```python
from build123d import *
from build123d.topology import SkipClean

# Parameters (mm, degrees)
SKETCH2_W                      = 63.5
SKETCH2_H                      = 63.5
BOSS_EXTRUDE1_DEPTH            = 80
CUT_EXTRUDE1_REACH             = 93.739
SKETCH4_R                      = 14.2875
CUT_EXTRUDE2_DEPTH             = 3.81
CUT_EXTRUDE3_DEPTH             = 62.22
CUT_EXTRUDE4_REACH             = 93.739
CUT_EXTRUDE4_DIRECTION_2_REACH = 93.739
FILLET2_R                      = 2.54
SKETCH9_W                      = 5
SKETCH9_H                      = 80
BOSS_EXTRUDE2_DEPTH            = 35
SKETCH10_R                     = 2.75
CUT_EXTRUDE6_DEPTH             = 119.642846392
CUT_EXTRUDE7_REACH             = 110.92
SKETCH11_R                     = 3
SKETCH12_W                     = 40
SKETCH12_H                     = 80
BOSS_EXTRUDE3_DEPTH            = 15
SKETCH13_R                     = 3
CUT_EXTRUDE8_DEPTH             = 10
FILLET3_R                      = 3.175
FILLET4_DEPTH                  = 80


with BuildPart() as part:
    # Sketch2 → Boss-Extrude1 (new body)
    with BuildSketch(Plane(origin=(0, 0, 0), x_dir=(1, 0, 0), z_dir=(0, 1, 0))):
        Rectangle(SKETCH2_W, SKETCH2_H)
    extrude(amount=BOSS_EXTRUDE1_DEPTH)

    # Sketch3 → Cut-Extrude1 (cut, up to next)
    with BuildSketch(Plane(origin=(0, 80, 0), x_dir=(1, 0, 0), z_dir=(0, 1, 0)), mode=Mode.PRIVATE) as cut_extrude1_sk1:
        with BuildLine():
            Line((9.525, 0), (14.2875, 0))
            ThreePointArc((14.2875, 0), (0, -14.2875), (-14.2875, 0))
            Line((-14.2875, 0), (-9.525, 0))
            ThreePointArc((-9.525, 0), (0, 9.525), (9.525, 0))
        make_face()
    cut_extrude1_tool1 = extrude(cut_extrude1_sk1.sketch, amount=-CUT_EXTRUDE1_REACH, mode=Mode.PRIVATE) & part.part
    add(cut_extrude1_tool1.solids().sort_by_distance((0, 80, 2.954161))[0], mode=Mode.SUBTRACT)

    # Sketch4 → Cut-Extrude2 (cut)
    with BuildSketch(Plane(origin=(0, 80, 0), x_dir=(1, 0, 0), z_dir=(0, 1, 0))):
        with Locations(Location((0, 0, 0), (0, 0, 270))):
            Circle(SKETCH4_R)
    extrude(amount=-CUT_EXTRUDE2_DEPTH, mode=Mode.SUBTRACT)

    # Sketch6 → Cut-Extrude3 (cut)
    with BuildSketch(Plane(origin=(0, 71.11, 0), x_dir=(1, 0, 0), z_dir=(0, 1, 0))):
        with BuildLine():
            Line((9.525, 0), (19.05, 31.75))
            Line((19.05, 31.75), (-19.05, 31.75))
            Line((-19.05, 31.75), (-9.525, 0))
            ThreePointArc((-9.525, 0), (0, 9.525), (9.525, 0))
        make_face()
    extrude(amount=-CUT_EXTRUDE3_DEPTH, mode=Mode.SUBTRACT)

    # Cut-Extrude4: up to this plane
    with SkipClean():  # the faces are left unmerged after this step: merging them gives an invalid solid
        cut_extrude4_end = Plane(origin=(-9.525, -49.595085442, 0), z_dir=(-0.9578262852211514, 0, 0.2873478855663456))
        # Sketch7 → Cut-Extrude4 (cut, up to the surface)
        with BuildSketch(Plane(origin=(0, 0, 0), x_dir=(0, 0, -1), z_dir=(1, 0, 0)), mode=Mode.PRIVATE) as cut_extrude4_sk1:
            Polygon((0, 8.89), (31.75, 8.89), (0, 0), align=None)
        cut_extrude4_tool1 = split(extrude(cut_extrude4_sk1.sketch, amount=-CUT_EXTRUDE4_REACH, mode=Mode.PRIVATE), bisect_by=cut_extrude4_end, keep=Keep.BOTH, mode=Mode.PRIVATE)
        add(cut_extrude4_tool1.solids().sort_by_distance((0, 5.926667, -10.583333))[0], mode=Mode.SUBTRACT)

    # Cut-Extrude4 direction 2: up to this plane
    cut_extrude4_direction_2_end = Plane(origin=(9.525, -49.595085442, 0), z_dir=(0.9578262852211514, 0, 0.2873478855663456))
    # Sketch7 → Cut-Extrude4 direction 2 (cut, up to the surface)
    with BuildSketch(Plane(origin=(0, 0, 0), x_dir=(0, 0, -1), z_dir=(1, 0, 0)), mode=Mode.PRIVATE) as cut_extrude4_direction_2_sk1:
        Polygon((0, 8.89), (31.75, 8.89), (0, 0), align=None)
    cut_extrude4_direction_2_tool1 = split(extrude(cut_extrude4_direction_2_sk1.sketch, amount=CUT_EXTRUDE4_DIRECTION_2_REACH, mode=Mode.PRIVATE), bisect_by=cut_extrude4_direction_2_end, keep=Keep.BOTH, mode=Mode.PRIVATE)
    add(cut_extrude4_direction_2_tool1.solids().sort_by_distance((0, 5.926667, -10.583333))[0], mode=Mode.SUBTRACT)

    # Fillet2
    # the kernel refuses this fillet: 2.54 mm, written as the material it adds along each edge
    with BuildSketch(Plane(origin=(7.700340927, 71.11, 6.082196911), x_dir=(-0.9578262852211513, 0, -0.2873478855663455), z_dir=(0.28734788556634555, 0, -0.9578262852211513))) as fillet2_piece_1_section:
        with BuildLine():
            CenterArc((FILLET2_R, -FILLET2_R), FILLET2_R, 90, 90)
            Line((0, -FILLET2_R), (0, 0))
            Line((0, 0), (FILLET2_R, 0))
        make_face()
    fillet2_piece_1 = extrude(amount=45.847973166, mode=Mode.PRIVATE)
    fillet2_piece_1 = split(fillet2_piece_1, bisect_by=Plane(origin=(7.700340927, 71.11, -31.75), z_dir=(0, 0, 1)), keep=Keep.TOP, mode=Mode.PRIVATE)
    fillet2_piece_1 = fillet2_piece_1 - Plane(origin=(0, 71.11, 0), x_dir=(-1, 0, 0), z_dir=(0, 1, 0)) * Cylinder(9.525, 102, mode=Mode.PRIVATE)
    fillet2_piece_1 = split(fillet2_piece_1, bisect_by=Plane(origin=(7.700340927, 71.11, 0), z_dir=(0, 0, -1)), keep=Keep.TOP, mode=Mode.PRIVATE)
    add(fillet2_piece_1)
    with BuildSketch(Plane(origin=(-20.874659073, 71.11, -37.832196911), x_dir=(0, -1, 0), z_dir=(0.28734788556634555, 0, 0.9578262852211513))) as fillet2_piece_2_section:
        with BuildLine():
            CenterArc((FILLET2_R, FILLET2_R), FILLET2_R, 180, 90)
            Line((0, FILLET2_R), (0, 0))
            Line((0, 0), (FILLET2_R, 0))
        make_face()
    fillet2_piece_2 = extrude(amount=45.847973166, mode=Mode.PRIVATE)
    fillet2_piece_2 = split(fillet2_piece_2, bisect_by=Plane(origin=(-20.874659073, 71.11, -31.75), z_dir=(0, 0, 1)), keep=Keep.TOP, mode=Mode.PRIVATE)
    fillet2_piece_2 = split(fillet2_piece_2, bisect_by=Plane(origin=(-20.874659073, 71.11, 0), z_dir=(0, 0, -1)), keep=Keep.TOP, mode=Mode.PRIVATE)
    fillet2_piece_2 = fillet2_piece_2 - Plane(origin=(0, 71.11, 0), x_dir=(-1, 0, 0), z_dir=(0, 1, 0)) * Cylinder(9.525, 102, mode=Mode.PRIVATE)
    add(fillet2_piece_2)
    with BuildSketch(Plane(origin=(-20.954648619, 10.667672044, -38.098828729), x_dir=(0.9607141016314922, 0.07483307171461691, -0.2672609704093551), z_dir=(0.2775399339309484, -0.2590372716688848, 0.9251331131031606))) as fillet2_piece_3_section:
        with BuildLine():
            CenterArc((FILLET2_R * 1.08072615035, FILLET2_R), FILLET2_R, 175.556407911, 94.443592089)
            Line((FILLET2_R * 0.0837320564804, FILLET2_R * 1.07747758898), (0, 0))
            Line((0, 0), (FILLET2_R * 1.08072615035, 0))
        make_face()
    fillet2_piece_3 = extrude(amount=52.848435405, mode=Mode.PRIVATE)
    fillet2_piece_3 = split(fillet2_piece_3, bisect_by=Plane(origin=(-20.954648619, 10.667672044, -31.75), z_dir=(0, 0, 1)), keep=Keep.TOP, mode=Mode.PRIVATE)
    fillet2_piece_3 = fillet2_piece_3 - Plane(origin=(0, 10.667672044, 0), x_dir=(-1, 0, 0), z_dir=(0, 1, 0)) * Cylinder(9.525, 117, mode=Mode.PRIVATE)
    fillet2_piece_3 = split(fillet2_piece_3, bisect_by=Plane(origin=(-20.954648619, 10.667672044, 0), z_dir=(0, 0, -1)), keep=Keep.TOP, mode=Mode.PRIVATE)
    add(fillet2_piece_3)
    with BuildSketch(Plane(origin=(20.954648619, 10.667672044, -38.098828729), x_dir=(-0.9607141016314922, 0.07483307171461691, -0.2672609704093551), z_dir=(-0.2775399339309484, -0.2590372716688848, 0.9251331131031606))) as fillet2_piece_4_section:
        with BuildLine():
            CenterArc((FILLET2_R * 1.08072615035, -FILLET2_R), FILLET2_R, 90, 94.443592089)
            Line((FILLET2_R * 0.0837320564804, -FILLET2_R * 1.07747758898), (0, 0))
            Line((0, 0), (FILLET2_R * 1.08072615035, 0))
        make_face()
    fillet2_piece_4 = extrude(amount=52.848435405, mode=Mode.PRIVATE)
    fillet2_piece_4 = split(fillet2_piece_4, bisect_by=Plane(origin=(20.954648619, 10.667672044, -31.75), z_dir=(0, 0, 1)), keep=Keep.TOP, mode=Mode.PRIVATE)
    fillet2_piece_4 = fillet2_piece_4 - Plane(origin=(0, 10.667672044, 0), x_dir=(-1, 0, 0), z_dir=(0, 1, 0)) * Cylinder(9.525, 117, mode=Mode.PRIVATE)
    fillet2_piece_4 = split(fillet2_piece_4, bisect_by=Plane(origin=(20.954648619, 10.667672044, 0), z_dir=(0, 0, -1)), keep=Keep.TOP, mode=Mode.PRIVATE)
    add(fillet2_piece_4)

    # Sketch9 → Boss-Extrude2 (add)
    with BuildSketch(Plane.XY.offset(31.75)):
        with Locations((-22.5, 40)):
            Rectangle(SKETCH9_W, SKETCH9_H)
        with Locations((22.5, 40)):
            Rectangle(SKETCH9_W, SKETCH9_H)
    extrude(amount=BOSS_EXTRUDE2_DEPTH)

    # Sketch10 → Cut-Extrude6 (cut, through all)
    with BuildSketch(Plane.ZY.offset(25)):
        with Locations(Location((56.75, 70, 0), (0, 0, 270))):
            Circle(SKETCH10_R)
        with Locations(Location((56.75, 10, 0), (0, 0, 270))):
            Circle(SKETCH10_R)
    extrude(amount=-CUT_EXTRUDE6_DEPTH, mode=Mode.SUBTRACT)

    # Sketch11 → Cut-Extrude7 (cut, up to next)
    with BuildSketch(Plane.XZ, mode=Mode.PRIVATE) as cut_extrude7_sk1:
        with Locations(Location((26.042742751, -26.042742751, 0), (0, 0, 270))):
            Circle(SKETCH11_R)
    cut_extrude7_tool1 = extrude(cut_extrude7_sk1.sketch, amount=-CUT_EXTRUDE7_REACH, mode=Mode.PRIVATE) & part.part
    # Sketch11 → Cut-Extrude7 (cut, up to next)
    with BuildSketch(Plane.XZ, mode=Mode.PRIVATE) as cut_extrude7_sk2:
        with Locations(Location((26.042742751, 26.042742751, 0), (0, 0, 270))):
            Circle(SKETCH11_R)
    cut_extrude7_tool2 = extrude(cut_extrude7_sk2.sketch, amount=-CUT_EXTRUDE7_REACH, mode=Mode.PRIVATE) & part.part
    # Sketch11 → Cut-Extrude7 (cut, up to next)
    with BuildSketch(Plane.XZ, mode=Mode.PRIVATE) as cut_extrude7_sk3:
        with Locations(Location((-26.042742751, -26.042742751, 0), (0, 0, 270))):
            Circle(SKETCH11_R)
    cut_extrude7_tool3 = extrude(cut_extrude7_sk3.sketch, amount=-CUT_EXTRUDE7_REACH, mode=Mode.PRIVATE) & part.part
    # Sketch11 → Cut-Extrude7 (cut, up to next)
    with BuildSketch(Plane.XZ, mode=Mode.PRIVATE) as cut_extrude7_sk4:
        with Locations(Location((-26.042742751, 26.042742751, 0), (0, 0, 270))):
            Circle(SKETCH11_R)
    cut_extrude7_tool4 = extrude(cut_extrude7_sk4.sketch, amount=-CUT_EXTRUDE7_REACH, mode=Mode.PRIVATE) & part.part
    add(cut_extrude7_tool1.solids().sort_by_distance((26.042743, 0, -26.042743))[0], mode=Mode.SUBTRACT)
    add(cut_extrude7_tool2.solids().sort_by_distance((26.042743, 0, 26.042743))[0], mode=Mode.SUBTRACT)
    add(cut_extrude7_tool3.solids().sort_by_distance((-26.042743, 0, -26.042743))[0], mode=Mode.SUBTRACT)
    add(cut_extrude7_tool4.solids().sort_by_distance((-26.042743, 0, 26.042743))[0], mode=Mode.SUBTRACT)

    # Sketch12 → Boss-Extrude3 (add)
    with BuildSketch(Plane.XY.offset(31.75)):
        with Locations((0, 40)):
            Rectangle(SKETCH12_W, SKETCH12_H)
    extrude(amount=BOSS_EXTRUDE3_DEPTH)

    # Sketch13 → Cut-Extrude8 (cut)
    with BuildSketch(Plane(origin=(0, 0, -31.75), x_dir=(-1, 0, 0), z_dir=(0, 0, -1))):
        with Locations((-18.75, 75)):
            Circle(SKETCH13_R)
        with Locations(Location((18.75, 75, 0), (0, 0, 180))):
            Circle(SKETCH13_R)
        with Locations((18.75, 5)):
            Circle(SKETCH13_R)
        with Locations(Location((-18.75, 5, 0), (0, 0, 180))):
            Circle(SKETCH13_R)
    extrude(amount=-CUT_EXTRUDE8_DEPTH, mode=Mode.SUBTRACT)

    # Fillet3
    fillet3_edges = [part.edges().sort_by_distance(p)[0] for p in [
        (31.75, 40, 31.75),
        (-31.75, 40, 31.75),
        (-31.75, 40, -31.75),
        (31.75, 40, -31.75),
    ]]
    fillet(fillet3_edges, radius=FILLET3_R)

    # Fillet4: read off the stored shape, not the designer's step
    # Fillet4 outline → Fillet4 (add)
    with BuildSketch(Plane(origin=(0, 0, 0), x_dir=(1, 0, 0), z_dir=(0, 1, 0))):
        with BuildLine():
            Line((25, -31.75), (25, -36.624844719))
            ThreePointArc((25, -36.624844719), (26.168694859, -33.412197692), (29.128440367, -31.701392291))
            ThreePointArc((29.128440367, -31.701392291), (28.852785416, -31.737824728), (28.575, -31.75))
            Line((28.575, -31.75), (25, -31.75))
        make_face()
        with BuildLine():
            ThreePointArc((-28.575, -31.75), (-28.852785416, -31.737824728), (-29.128440367, -31.701392291))
            ThreePointArc((-29.128440367, -31.701392291), (-26.168694859, -33.412197692), (-25, -36.624844719))
            Line((-25, -36.624844719), (-25, -31.75))
            Line((-25, -31.75), (-28.575, -31.75))
        make_face()
    extrude(amount=FILLET4_DEPTH)


solid = part.part
```
The listing builds one solid part. Answer for the finished solid, in the listing's coordinates (mm). A direction names the side the tool comes from. Coordinates: 2 decimals unless noted, no trailing zeros. Write each loop counter-clockwise with the first axis right and the second up, starting at its lowest first coordinate (ties: lowest second). Pieces come first, ordered by that corner, then holes.
Q1. The mould has two halves that part along X. Classify faces 6 (the cylindrical face through (26.137, 39.44, 33.45)), 7 (the flat face through (-23, 41, 66.75)), 8 (the flat face through (19, 75, -21.75)), 9 (the cylindrical face through (-31.03, 40.56, 30.59)): released by +X, released by -X, zero draft, split by the parting line, or undercut.
Returned:
face 6: released by +X
face 7: zero draft
face 8: undercut
face 9: released by -X
Q2. Section D-D, the plane z = 43.5 is taken. Write down the section's boundary in (x, y).
Returned:
outline: (-25, 0) - (25, 0) - (25, 80) - (-25, 80) - close
Q3. Find the intervals of material crossed by line 1 along Y through (x, z) = (18.75, -28.75); line 2 along Z through (x, y) = (-23, 10); line 3 along Z through (x, y) = (-24.5, 47.5), in increasing order.
Returned:
line 1: y = 0 to 2, 8 to 72, 78 to 80
line 2: z = -31.75 to 54, 59.5 to 66.75
line 3: z = -31.75 to -28.62, -23.47 to 23.47, 28.62 to 66.75
Q4. Given P1, Ø6, axis at y = 35, z = 54.5, coming from the +X side; P2, Ø5, axis at x = -26.04, z = -26.04, coming from the +Y side; P3, Ø1.4, axis at x = -12.5, y = 24.5, coming from the +Z side; P4, Ø3, axis at x = 18, y = 74.5, coming from the -Z side, each flat-ended and moving along its own axis, determine where each tip first touches the part or whether it passes through.
Returned:
P1: stops at x = 25
P2: passes through
P3: stops at z = 46.75
P4: stops at z = -21.75
Q5. Section B-B, the plane y = 47.5 is taken. Give the number of separate pieces and of enclosed holes in the cut face, then the cut area to 3 significant figures.
Returned:
separate pieces: 1
enclosed holes: 4
area: 3,640 mm2
Q6. Section A-A, the plane z = 56.75 is taken. Write down the section's boundary in (x, y), then the cut area to 3 significant figures.
Returned:
outline: (-25, 0) - (-20, 0) - (-20, 7.25) - (-25, 7.25) - close; (-25, 12.75) - (-20, 12.75) - (-20, 67.25) - (-25, 67.25) - close; (-25, 72.75) - (-20, 72.75) - (-20, 80) - (-25, 80) - close; (20, 0) - (25, 0) - (25, 7.25) - (20, 7.25) - close; (20, 12.75) - (25, 12.75) - (25, 67.25) - (20, 67.25) - close; (20, 72.75) - (25, 72.75) - (25, 80) - (20, 80) - close
area: 690 mm2
Q7. Which of the six approach directions +Z, -Z, +X, -X, +Y, -Y give full straight-line access (tool end or side, diameter ignored) to faces 1 (the cylindrical face through (-13.6, 70.4, -16.3)), 2 (the flat face through (22, 41, 66.75)), 3 (the flat face through (0, 76.19, -10)), 4 (the flat face through (-0.227, 6.023, -21.509)), 5 (the cylindrical face through (-25.142, 39.44, -28.904))?
Returned:
face 1: -Z
face 2: +Z, +X, -X, +Y, -Y
face 3: +Y
face 4: none
face 5: +Y, -Y
